```python
from build123d import *

# Parameters (mm, degrees)
BOX009_W                    = 20
BOX009_H                    = 2
BOX009_DEPTH                = 80
BOX010_W                    = 20
BOX010_H                    = 2
BOX010_DEPTH                = 80
COMPOUND004_PLACEMENT_ANGLE = 90
TUBE012_R                   = 10
TUBE012_R_2                 = 3.25
TUBE012_DEPTH               = 80
CYLINDER003_R               = 1.7
CYLINDER003_DEPTH           = 12
CYLINDER004_R               = 3.25
CYLINDER004_DEPTH           = 9
CYLINDER005_R               = 1.7
CYLINDER005_DEPTH           = 12
CYLINDER006_R               = 3.25
CYLINDER006_DEPTH           = 9
TUBE005_R                   = 7.625
TUBE005_R_2                 = 5.625
TUBE005_DEPTH               = 5
TUBE004_R                   = 7.625
TUBE004_R_2                 = 5.625
TUBE004_DEPTH               = 5
BOX003_W                    = 20
BOX003_H                    = 0.5
BOX003_DEPTH                = 40
BOX004_W                    = 20
BOX004_H                    = 0.5
BOX004_DEPTH                = 40
COMPOUND001_PLACEMENT_ANGLE = 90
TUBE003_R                   = 10
TUBE003_R_2                 = 3.25
TUBE003_DEPTH               = 40
CYLINDER_R                  = 5.625
CYLINDER_DEPTH              = 100
BOX002_W                    = 23
BOX002_H                    = 42
BOX002_DEPTH                = 12


with BuildPart() as cube009:
    # Box009 → Box009 (new body)
    with BuildSketch(Plane(origin=(-10, -1, -20), x_dir=(1, 0, 0), z_dir=(0, 0, 1))):
        with Locations((10, 1)):
            Rectangle(BOX009_W, BOX009_H)
    extrude(amount=BOX009_DEPTH)


with BuildPart() as fusion007:
    # Box010 → Box010 (new body)
    with BuildSketch(Plane(origin=(-10, -1, -20), x_dir=(1, 0, 0), z_dir=(0, 0, 1))):
        with Locations((10, 1)):
            Rectangle(BOX010_W, BOX010_H)
    extrude(amount=BOX010_DEPTH)


with BuildPart() as fusion007_1:
    # Compound004 placement: moved
    add(fusion007.part.rotate(Axis((0, 0, 0), (0, 0, 1)), COMPOUND004_PLACEMENT_ANGLE))

    # Fusion007: union Cube009
    add(cube009.part)


with BuildPart() as cut017:
    # Tube012 → Tube012 (new body)
    with BuildSketch(Plane.XY.offset(-20)):
        Circle(TUBE012_R)
        Circle(TUBE012_R_2, mode=Mode.SUBTRACT)
    extrude(amount=TUBE012_DEPTH)

    # Cut017: cut Fusion007
    add(fusion007_1.part, mode=Mode.SUBTRACT)


with BuildPart() as cylinder003:
    # Cylinder003 → Cylinder003 (new body)
    with BuildSketch(Plane.XY):
        Circle(CYLINDER003_R)
    extrude(amount=CYLINDER003_DEPTH)


with BuildPart() as fusion003:
    # Cylinder004 → Cylinder004 (new body)
    with BuildSketch(Plane.XY.offset(3)):
        Circle(CYLINDER004_R)
    extrude(amount=CYLINDER004_DEPTH)

    # Fusion003: union Cylinder003
    add(cylinder003.part)


with BuildPart() as fusion003_1:
    # Fusion003 placement: moved
    add(fusion003.part.moved(Location((-7.5, 18.5, 0))))


with BuildPart() as cylinder005:
    # Cylinder005 → Cylinder005 (new body)
    with BuildSketch(Plane.XY):
        Circle(CYLINDER005_R)
    extrude(amount=CYLINDER005_DEPTH)


with BuildPart() as fusion005:
    # Cylinder006 → Cylinder006 (new body)
    with BuildSketch(Plane.XY.offset(3)):
        Circle(CYLINDER006_R)
    extrude(amount=CYLINDER006_DEPTH)

    # Fusion004: union Cylinder005
    add(cylinder005.part)


with BuildPart() as fusion005_1:
    # Fusion004 placement: moved
    add(fusion005.part.moved(Location((-7.5, -18.5, 0))))

    # Fusion005: union Fusion003
    add(fusion003_1.part)


with BuildPart() as fusion005_2:
    # Fusion005 placement: moved
    add(fusion005_1.part.moved(Location((0, 0, 1))))


with BuildPart() as mountringgroove003:
    # Tube005 → Tube005 (new body)
    with BuildSketch(Plane.XY.offset(35)):
        Circle(TUBE005_R)
        Circle(TUBE005_R_2, mode=Mode.SUBTRACT)
    extrude(amount=TUBE005_DEPTH)


with BuildPart() as mountringgroove002:
    # Tube004 → Tube004 (new body)
    with BuildSketch(Plane.XY):
        Circle(TUBE004_R)
        Circle(TUBE004_R_2, mode=Mode.SUBTRACT)
    extrude(amount=TUBE004_DEPTH)


with BuildPart() as cube003:
    # Box003 → Box003 (new body)
    with BuildSketch(Plane(origin=(-10, -0.25, 0), x_dir=(1, 0, 0), z_dir=(0, 0, 1))):
        with Locations((10, 0.25)):
            Rectangle(BOX003_W, BOX003_H)
    extrude(amount=BOX003_DEPTH)


with BuildPart() as fusion001:
    # Box004 → Box004 (new body)
    with BuildSketch(Plane(origin=(-10, -0.25, 0), x_dir=(1, 0, 0), z_dir=(0, 0, 1))):
        with Locations((10, 0.25)):
            Rectangle(BOX004_W, BOX004_H)
    extrude(amount=BOX004_DEPTH)


with BuildPart() as fusion001_1:
    # Compound001 placement: moved
    add(fusion001.part.rotate(Axis((0, 0, 0), (0, 0, 1)), COMPOUND001_PLACEMENT_ANGLE))

    # Fusion001: union Cube003
    add(cube003.part)


with BuildPart() as cut006:
    # Tube003 → Tube003 (new body)
    with BuildSketch(Plane.XY):
        Circle(TUBE003_R)
        Circle(TUBE003_R_2, mode=Mode.SUBTRACT)
    extrude(amount=TUBE003_DEPTH)

    # Cut004: cut Fusion001
    add(fusion001_1.part, mode=Mode.SUBTRACT)

    # Cut005: cut MountringGroove002
    add(mountringgroove002.part, mode=Mode.SUBTRACT)

    # Cut006: cut MountringGroove003
    add(mountringgroove003.part, mode=Mode.SUBTRACT)


with BuildPart() as cut006_1:
    # Cut006 placement: moved
    add(cut006.part.moved(Location((0, 0, 7))))


with BuildPart() as cylinder:
    # Cylinder → Cylinder (new body)
    with BuildSketch(Plane.XY):
        Circle(CYLINDER_R)
    extrude(amount=CYLINDER_DEPTH)


with BuildPart() as bottommount:
    # Box002 → Box002 (new body)
    with BuildSketch(Plane(origin=(-11.5, -21, 0), x_dir=(1, 0, 0), z_dir=(0, 0, 1))):
        with Locations((11.5, 21)):
            Rectangle(BOX002_W, BOX002_H)
    extrude(amount=BOX002_DEPTH)

    # Cut003: cut Cylinder
    add(cylinder.part, mode=Mode.SUBTRACT)

    # Cut007: cut Cut006
    add(cut006_1.part, mode=Mode.SUBTRACT)


with BuildPart() as bottommount_1:
    # Cut007 placement: moved
    add(bottommount.part.moved(Location((0, 0, 1))))

    # Cut013: cut Fusion005
    add(fusion005_2.part, mode=Mode.SUBTRACT)


with BuildPart() as bottommount_2:
    # Cut013 placement: moved
    add(bottommount_1.part.moved(Location((0, 0, 4))))

    # Cut020: cut Cut017
    add(cut017.part, mode=Mode.SUBTRACT)


solid = bottommount_2.part
```
Geometry check sheet. Reference: the model listing, model coordinates, mm. A direction names the side the tool comes from. Give positions to 0.01 mm unless a question says otherwise; leave off trailing zeros. Write each loop counter-clockwise with the first axis right and the second up, starting at its lowest first coordinate (ties: lowest second). Pieces come first, ordered by that corner, then holes. Notation, with made-up numbers: (63, 0) -> (99, 0) arc R4 cw to (99, 7) -> close; hole circle Ø6 at (-13, 29.25). An arc over 180 degrees is marked (long way). One line per question, with ' | ' between items.
Item 1: Sectioned sample at C-C, the plane x = 3.25. Record the boundary of the cut face in (y, z), plus the area to 3 significant figures.
Determined:
outline: (-21, 5) -> (-9.46, 5) -> (-9.46, 17) -> (-21, 17) -> close; (9.46, 5) -> (21, 5) -> (21, 17) -> (9.46, 17) -> close | area: 277 mm^2
Item 2: Depth check by flat-ended pin: pin 1 (1.2 mm diameter, centred on x = -8.5, z = 14, fed in from +Y); pin 2 (0.6 mm diameter, centred on x = -9, y = -1, fed in from +Z); pin 3 (3 mm diameter, centred on x = -8.5, y = 18.5, fed in from +Z); pin 4 (2.5 mm diameter, centred on x = -7.5, y = 18.5, fed in from -Z). Enter the tip coordinate at first touch or a pass-through.
Determined:
pin 1: y = 15.67 | pin 2: z = 12 | pin 3: z = 8 | pin 4: through
Item 3: Sectioned sample at D-D, the plane y = -9. Record the boundary of the cut face in (x, z).
Determined:
outline: (-11.5, 5) -> (-4.36, 5) -> (-4.36, 17) -> (-11.5, 17) -> close; (-1, 5) -> (1, 5) -> (1, 12) -> (0.25, 12) -> (0.25, 17) -> (-0.25, 17) -> (-0.25, 12) -> (-1, 12) -> close; (4.36, 5) -> (11.5, 5) -> (11.5, 17) -> (4.36, 17) -> close
Item 4: Sectioned sample at B-B, the plane z = 6.5. Record the boundary of the cut face in (x, y) (3 decimals).
Determined:
outline: (-11.5, -21) -> (11.5, -21) -> (11.5, 21) -> (-11.5, 21) -> close; hole (-9.95, -1) arc R10 ccw to (-1, -9.95) -> (-1, -5.535) arc R5.625 ccw to (1, -5.535) -> (1, -9.95) arc R10 ccw to (9.95, -1) -> (5.535, -1) arc R5.625 ccw to (5.535, 1) -> (9.95, 1) arc R10 ccw to (1, 9.95) -> (1, 5.535) arc R5.625 ccw to (-1, 5.535) -> (-1, 9.95) arc R10 ccw to (-9.95, 1) -> (-5.535, 1) arc R5.625 ccw to (-5.535, -1) -> close; hole circle Ø3.4 at (-7.5, -18.5); hole circle Ø3.4 at (-7.5, 18.5)
Item 5: Draft check along Y on faces 1 (the flat face through (8, 0, 5)), 2 (the flat face through (0, 21, 11)), 3 (the flat face through (-0.25, 9, 14)). Enter one of: released by +Y, released by -Y, zero draft, split by the parting line, or undercut.
Determined:
face 1: zero draft | face 2: released by +Y | face 3: undercut
Item 6: Access from +Z, -Z, +X, -X, +Y, -Y to the whole of each face (thin tool, end or side, straight path). Record for faces 4 (the flat face through (7, -1, 10)), 5 (the flat face through (-9, -0.25, 14)), 6 (the flat face through (-11.5, 0, 11)).
Determined:
face 4: +Z, -Z | face 5: +Z | face 6: +Z, -Z, -X, +Y, -Y
Item 7: Scan lines: line 1 along X through (y, z) = (18.5, 5.8); line 2 along X through (y, z) = (0, 16.5) (3 decimals); line 3 along Y through (x, z) = (6, 7.5). Record each from-to range of solid material in increasing order.
Determined:
line 1: -11.5 to -9.2, -5.8 to 11.5 | line 2: -11.5 to -5.625, 5.625 to 11.5 | line 3: -21 to -8, -1 to 1, 8 to 21
Item 8: Sectioned sample at A-A, the plane y = -18.5. Record the boundary of the cut face in (x, z).
Determined:
outline: (-11.5, 5) -> (-9.2, 5) -> (-9.2, 8) -> (-10.75, 8) -> (-10.75, 17) -> (-11.5, 17) -> close; (-5.8, 5) -> (11.5, 5) -> (11.5, 17) -> (-4.25, 17) -> (-4.25, 8) -> (-5.8, 8) -> close
